from build123d import *

# Parameters (mm, degrees)
SKETCH_1_W          = 24
SKETCH_1_H          = 7
EXTRUDE_2_DEPTH     = 3
SKETCH_3_W          = 10
SKETCH_3_H          = 7
EXTRUDE_4_DEPTH     = 52
SKETCH_5_R          = 2.125
CUT_EXTRUDE_1_DEPTH = 7
SKETCH_6_R          = 1.5
CUT_EXTRUDE_2_DEPTH = 3
SKETCH_7_R          = 1.5
CUT_EXTRUDE_3_DEPTH = 3


with BuildPart() as part:
    # Эскиз1 → Бобышка-Вытянуть2 (new body)
    with BuildSketch(Plane.XY):
        Rectangle(SKETCH_1_W, SKETCH_1_H)
    extrude(amount=EXTRUDE_2_DEPTH)

    # Эскиз3 → Бобышка-Вытянуть4 (add)
    with BuildSketch(Plane.XY.offset(3)):
        Rectangle(SKETCH_3_W, SKETCH_3_H)
    extrude(amount=EXTRUDE_4_DEPTH)

    # Эскиз5 → Вырез-Вытянуть1 (cut)
    with BuildSketch(Plane(origin=(0, -3.5, 0), x_dir=(-1, 0, 0), z_dir=(0, -1, 0))):
        with Locations((0, -50)):
            Circle(SKETCH_5_R)
    extrude(amount=-CUT_EXTRUDE_1_DEPTH, mode=Mode.SUBTRACT)

    # Эскиз6 → Вырез-Вытянуть2 (cut)
    with BuildSketch(Plane.XY.offset(3)):
        with Locations((8.516484568, 0)):
            Circle(SKETCH_6_R)
    extrude(amount=-CUT_EXTRUDE_2_DEPTH, mode=Mode.SUBTRACT)

    # Эскиз7 → Вырез-Вытянуть3 (cut)
    with BuildSketch(Plane.XY.offset(3)):
        with Locations((-8.452342131, 0)):
            Circle(SKETCH_7_R)
    extrude(amount=-CUT_EXTRUDE_3_DEPTH, mode=Mode.SUBTRACT)


solid = part.part
Could you check a few things on this model? Use its own coordinates, in mm. A direction names the side the tool comes from. Give positions to 0.01 mm unless a question says otherwise; leave off trailing zeros. Order: outer loops, then holes, each group sorted by start corner. A loop starts at its lowest first (then second) coordinate and runs counter-clockwise, first axis right, second up. Notation, with made-up numbers: (12.5, -33.75) -> (19.5, -33.75) arc R13 cw to (19.5, -25.75) -> close; hole circle Ø4 at (-28, 32.5). An arc over 180 degrees is marked (long way). Answer in a Markdown table with one row per item. Add a question column.
Item 1: Please list where these lines run through material, in increasing order: probe 1 along Z at (x, y) = (0, -1) (3 decimals); probe 2 along X at (y, z) = (3, 47); probe 3 along Z at (x, y) = (-10, 3.25).
Item 2: I'm going to push flat-ended pins straight in: P1, Ø4, axis at x = 0, z = 50, coming from the -Y side; P2, Ø2, axis at y = 2, z = 22.5, coming from the -X side; P3, Ø2, axis at x = -8, y = -0.5, coming from the +Z side. Where does each tip first touch, or does it pass through?
Item 3: Imagine slicing it at C-C (x = 0). List the corners of the cut face in (y, z) for me (3 decimals), and give its area (3 significant figures).
Item 4: Imagine slicing it at A-A (y = 0). List the corners of the cut face in (x, z) for me (3 decimals).
Item 5: For faces 4 (the flat face through (5, 0, 29)), 5 (the flat face through (0, -3.5, 21)), 6 (the flat face through (-10.105, 0.049, 3)), which set-ups out of +Z, -Z, +X, -X, +Y, -Y let a thin tool reach every point of the face, with its end or its side?
Item 6: Imagine slicing it at B-B (z = 50). List the corners of the cut face in (x, y) for me (3 decimals).
Item 7: Imagine slicing it at D-D (y = -3). List the corners of the cut face in (x, z) for me (3 decimals).
Item 8: We'd pull the mould along Y, two halves only. Please class faces 1 (the cylindrical face through (-9.95, 0.07, 1.52)), 2 (the flat face through (-5, 0, 29)), 3 (the flat face through (0, 3.5, 21)): pulls with the +Y half, pulls with the -Y half, needs draft (parallel to the pull), parting line crosses it, or undercut.
Result:
| question | item | result |
|---|---|---|
| 1 | probe 1 | 0 to 47.875, 52.125 to 55 |
| 1 | probe 2 | -5 to 5 |
| 1 | probe 3 | 0 to 3 |
| 2 | P1 | through |
| 2 | P2 | x = -5 |
| 2 | P3 | z = 3 |
| 3 | outline | (-3.5, 0) -> (3.5, 0) -> (3.5, 47.875) -> (-3.5, 47.875) -> close; (-3.5, 52.125) -> (3.5, 52.125) -> (3.5, 55) -> (-3.5, 55) -> close |
| 3 | area | 355 mm2 |
| 4 | outline | (-12, 0) -> (-9.952, 0) -> (-9.952, 3) -> (-12, 3) -> close; (-6.952, 0) -> (7.016, 0) -> (7.016, 3) -> (5, 3) -> (5, 55) -> (-5, 55) -> (-5, 3) -> (-6.952, 3) -> close; (10.016, 0) -> (12, 0) -> (12, 3) -> (10.016, 3) -> close; hole circle Ø4.25 at (0, 50) |
| 5 | face 4 | +Z, +X, +Y, -Y |
| 5 | face 5 | +Z, -Z, +X, -X, -Y |
| 5 | face 6 | +Z, -X, +Y, -Y |
| 6 | outline | (-5, -3.5) -> (-2.125, -3.5) -> (-2.125, 3.5) -> (-5, 3.5) -> close; (2.125, -3.5) -> (5, -3.5) -> (5, 3.5) -> (2.125, 3.5) -> close |
| 7 | outline | (-12, 0) -> (12, 0) -> (12, 3) -> (5, 3) -> (5, 55) -> (-5, 55) -> (-5, 3) -> (-12, 3) -> close; hole circle Ø4.25 at (0, 50) |
| 8 | face 1 | undercut |
| 8 | face 2 | needs draft |
| 8 | face 3 | pulls with the +Y half |
